The model under review builds one solid part; all positions refer to its coordinate system, in mm. Face numbers are marked on the shaded views. Coordinates: 2 decimals unless noted, no trailing zeros. Loops run counter-clockwise (first coordinate to the right, second up) from the corner with the lowest first, then second, coordinate; pieces in that order, holes last. Notation, with made-up numbers: (65, -33.5) - (115, -33.5) arc R19 ccw to (115, -24.5) - close; hole circle Ø5 at (-26, 5). An arc over 180 degrees is marked (long way). Use a Markdown table: item, result. Add a question column.
1) Add section C-C, the plane x = -156.5. Give the boundary of the cut face in (y, z).
2) The part is to be moulded in two halves that separate along Z. For the marked faces 1, 2 and 3, say which applies: pulls with the +Z half, pulls with the -Z half, needs draft (parallel to the pull), parting line crosses it, or undercut.
3) Clearance check with flat-ended pins moving along their axes: pin 1 (2 mm diameter, centred on x = -50.5, z = 56.5, fed in from +Y); pin 2 (1.5 mm diameter, centred on x = -16.5, y = 7, fed in from +Z); pin 3 (5 mm diameter, centred on y = 1, z = 7.5, fed in from -X). State where each tip first meets the part, or that it passes through.
4) Add section B-B, the plane x = 0. Give the boundary of the cut face in (y, z).
5) To check wall thickness, follow L1, parallel to X at y = -3.25, z = 86.6; L2, parallel to X at y = 0, z = 10; L3, parallel to Z at x = -7, y = 7.5. State the ranges of each line that lie inside material, in increasing order. Write a range as [from, to].
6) Add section A-A, the plane z = -86.6. Give the boundary of the cut face in (x, y).
7) Add section D-D, the plane z = 0. Give the boundary of the cut face in (x, y), and give its area (3 significant figures).
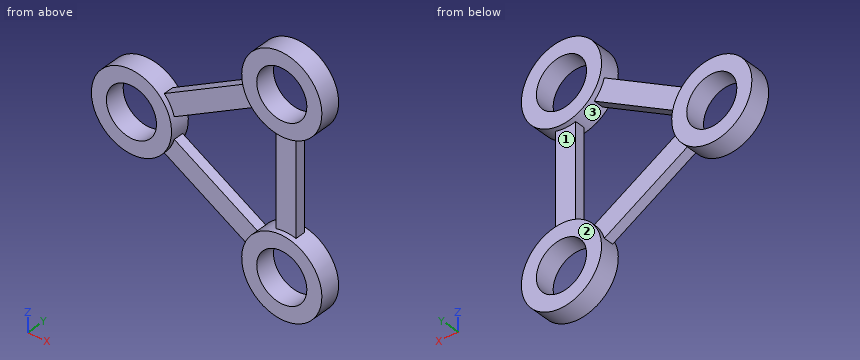
```python
from build123d import *

# Parameters (mm, degrees)
Y_KSEKLIK_EKSTR_ZYON4_DEPTH        = 10
Y_KSEKLIK_EKSTR_ZYON4_DEPTH_BACK   = 10
IZIM1_R                            = 40.003689591
IZIM1_R_2                          = 25
Y_KSEKLIK_EKSTR_ZYON4_2_DEPTH      = 10
Y_KSEKLIK_EKSTR_ZYON4_2_DEPTH_BACK = 10
IZIM1_R_3                          = 40
Y_KSEKLIK_EKSTR_ZYON4_3_DEPTH      = 10
Y_KSEKLIK_EKSTR_ZYON4_3_DEPTH_BACK = 10
Y_KSEKLIK_EKSTR_ZYON5_DEPTH        = 5
Y_KSEKLIK_EKSTR_ZYON5_DEPTH_BACK   = 5


with BuildPart() as part:
    # izim1 → Y_kseklik-Ekstr_zyon4 (new, two sides: drawn at the far end of the back side and taken through both)
    with BuildSketch(Plane(origin=(0, 0, 0), x_dir=(1, 0, 0), z_dir=(0, 1, 0)).offset(-Y_KSEKLIK_EKSTR_ZYON4_DEPTH_BACK)):
        with Locations(Location((-150, 0, 0), (0, 0, 270))):
            Circle(IZIM1_R)
        with Locations(Location((-150, 0, 0), (0, 0, 270))):
            Circle(IZIM1_R_2, mode=Mode.SUBTRACT)
    extrude(amount=Y_KSEKLIK_EKSTR_ZYON4_DEPTH + Y_KSEKLIK_EKSTR_ZYON4_DEPTH_BACK)



with BuildPart() as body_2:
    # izim1 → Y_kseklik-Ekstr_zyon4 2 (new, two sides: drawn at the far end of the back side and taken through both)
    with BuildSketch(Plane(origin=(0, 0, 0), x_dir=(1, 0, 0), z_dir=(0, 1, 0)).offset(-Y_KSEKLIK_EKSTR_ZYON4_2_DEPTH_BACK)):
        with Locations(Location((0, -86.6, 0), (0, 0, 270))):
            Circle(IZIM1_R_3)
        with Locations(Location((0, -86.6, 0), (0, 0, 270))):
            Circle(IZIM1_R_2, mode=Mode.SUBTRACT)
    extrude(amount=Y_KSEKLIK_EKSTR_ZYON4_2_DEPTH + Y_KSEKLIK_EKSTR_ZYON4_2_DEPTH_BACK)


with BuildPart() as body_3:
    # izim1 → Y_kseklik-Ekstr_zyon4 3 (new, two sides: drawn at the far end of the back side and taken through both)
    with BuildSketch(Plane(origin=(0, 0, 0), x_dir=(1, 0, 0), z_dir=(0, 1, 0)).offset(-Y_KSEKLIK_EKSTR_ZYON4_3_DEPTH_BACK)):
        with Locations(Location((0, 86.6, 0), (0, 0, 270))):
            Circle(IZIM1_R_3)
        with Locations(Location((0, 86.6, 0), (0, 0, 270))):
            Circle(IZIM1_R_2, mode=Mode.SUBTRACT)
    extrude(amount=Y_KSEKLIK_EKSTR_ZYON4_3_DEPTH + Y_KSEKLIK_EKSTR_ZYON4_3_DEPTH_BACK)


with BuildPart() as part_1:
    add(part.part)

    add(body_2.part)  # Y_kseklik-Ekstr_zyon5 merges body 2

    add(body_3.part)  # Y_kseklik-Ekstr_zyon5 merges body 3
    # izim1_6 → Y_kseklik-Ekstr_zyon5 (add, two sides: drawn at the far end of the back side and taken through both)
    with BuildSketch(Plane(origin=(0, 0, 0), x_dir=(1, 0, 0), z_dir=(0, 1, 0)).offset(-Y_KSEKLIK_EKSTR_ZYON5_DEPTH_BACK)):
        with BuildLine():
            ThreePointArc((-38.54115563, -75.895826855), (-34.641270188, -66.600440011), (-28.541375636, -58.575191761))
            Line((-28.541375636, -58.575191761), (-111.455544285, -10.706078394))
            ThreePointArc((-111.455544285, -10.706078394), (-115.355534509, -20.001404744), (-121.45532428, -28.026713488))
            Line((-121.45532428, -28.026713488), (-38.54115563, -75.895826855))
        make_face()
        with BuildLine():
            Line((-111.455544285, 10.706078394), (-28.541375636, 58.575191761))
            ThreePointArc((-28.541375636, 58.575191761), (-34.641270188, 66.600440011), (-38.54115563, 75.895826855))
            Line((-38.54115563, 75.895826855), (-121.45532428, 28.026713488))
            ThreePointArc((-121.45532428, 28.026713488), (-115.355534509, 20.001404744), (-111.455544285, 10.706078394))
        make_face()
        with BuildLine():
            ThreePointArc((10, 47.870166538), (0, 46.6), (-10, 47.870166538))
            Line((-10, 47.870166538), (-10, -47.870166538))
            ThreePointArc((-10, -47.870166538), (0, -46.6), (10, -47.870166538))
            Line((10, -47.870166538), (10, 47.870166538))
        make_face()
    extrude(amount=Y_KSEKLIK_EKSTR_ZYON5_DEPTH + Y_KSEKLIK_EKSTR_ZYON5_DEPTH_BACK)


solid = part_1.part
```
From the geometry:
| question | item | result |
|---|---|---|
| 1 | outline | (-10, -39.47) - (10, -39.47) - (10, -24.14) - (-10, -24.14) - close; (-10, 24.14) - (10, 24.14) - (10, 39.47) - (-10, 39.47) - close |
| 2 | face 1 | undercut |
| 2 | face 2 | needs draft |
| 2 | face 3 | undercut |
| 3 | pin 1 | stops at y = 5 |
| 3 | pin 2 | stops at z = 123.37 |
| 3 | pin 3 | stops at x = -189.69 |
| 4 | outline | (-10, -126.6) - (10, -126.6) - (10, -111.6) - (-10, -111.6) - close; (-10, -61.6) - (10, -61.6) - (10, -46.6) - (5, -46.6) - (5, 46.6) - (10, 46.6) - (10, 61.6) - (-10, 61.6) - (-10, 46.6) - (-5, 46.6) - (-5, -46.6) - (-10, -46.6) - close; (-10, 111.6) - (10, 111.6) - (10, 126.6) - (-10, 126.6) - close |
| 5 | L1 | x = [-40, -25], [25, 40] |
| 5 | L2 | x = [-188.73, -172.91], [-127.09, -111.27], [-10, 10] |
| 5 | L3 | z = [-125.98, -110.6], [-62.6, -47.22], [47.22, 62.6], [110.6, 125.98] |
| 6 | outline | (-40, -10) - (-25, -10) - (-25, 10) - (-40, 10) - close; (25, -10) - (40, -10) - (40, 10) - (25, 10) - close |
| 7 | outline | (-190, -10) - (-175, -10) - (-175, 10) - (-190, 10) - close; (-125, -10) - (-110, -10) - (-110, 10) - (-125, 10) - close; (-10, -5) - (10, -5) - (10, 5) - (-10, 5) - close |
| 7 | area | 800 mm^2 |
